Verification items for the finished model (mm, model axes). Face numbers are marked on the shaded views. A direction names the side the tool comes from. Coordinates: 2 decimals unless noted, no trailing zeros. Loops run counter-clockwise (first coordinate to the right, second up) from the corner with the lowest first, then second, coordinate; pieces in that order, holes last. Notation, with made-up numbers: (42, 22.25) -> (90, 22.25) arc R29 cw to (90, 49.25) -> close; hole circle Ø1 at (17, 56.25). An arc over 180 degrees is marked (long way). Answer as a JSON object with one key per item and string values. Group by question number.
Q1. Cross-section at B-B on y = 12.7. Record the boundary of the cut face in (x, z) (3 decimals).
Q2. Scan lines: L1, parallel to Z at x = 25.4, y = 28.15; L2, parallel to Z at x = 38.1, y = 29.15; L3, parallel to Y at x = 10.5, z = 23 (3 decimals). Record each from-to range of solid material in increasing order.
Q3. Set-up check for the marked faces 1 and 2: record each of +Z, -Z, +X, -X, +Y, -Y from which the full face is reachable in a straight line by a thin tool's end or side.
Q4. Cross-section at A-A on x = 6.35. Record the boundary of the cut face in (y, z) (3 decimals).
Q5. Cross-section at C-C on x = 25.4. Record the boundary of the cut face in (y, z) (3 decimals), and give its area (3 significant figures).
Q6. Gauge pin test, flat ends, axial feed: pin 1 Ø5.5 at (x, y) = (6.35, 12.7) entering from +Z (3 decimals); pin 2 Ø1.5 at (x, z) = (32.5, 45) entering from -Y. Record the tip position at first contact, or that the pin passes through.
Q7. Cross-section at D-D on x = 13. Record the boundary of the cut face in (y, z) (3 decimals).
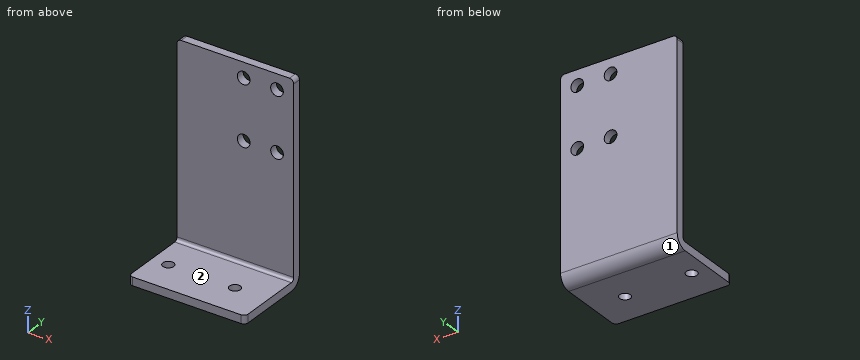
Autodesk Inventor part; units mm, degrees
ref_plane "YZ Plane" through (0, 0, 0) normal (1, 0, 0) x (0, 1, 0)
ref_plane "XZ Plane" through (0, 0, 0) normal (0, 1, 0) x (-1, 0, 0)
ref_plane "XY Plane" through (0, 0, 0) normal (0, 0, 1) x (1, 0, 0)
sketch "Sketch1" plane through (0, 0, 0) normal (0, 0, 1) x (1, 0, 0)
  line L0 (0, 0) -> (44.45, 0)
  line L1 (44.45, 0) -> (44.45, 25.4)
  line L2 (44.45, 25.4) -> (0, 25.4)
  line L3 (0, 25.4) -> (0, 0)
  circle A0 centre (6.35, 12.7) radius 2.0701
  line L4 (0, 12.7) -> (44.45, 12.7) construction
  circle A1 centre (31.75, 12.7) radius 2.0701
  dimension "d0" = 44.45
  dimension "d1" = 25.4
  dimension "d2" = 4.1402
  dimension "d6" = 25.4
  dimension "d34" = 6.35
extrude "Plate1" add sketch "Sketch1" along normal blind 3.175
sketch "Sketch2" plane through (0, 26.67, 4.445) normal (0, 1, 0) x (-1, 0, 0)
  line L0 (-44.45, 0) -> (0, 0)
  line L1 (0, 0) -> (0, 71.755)
  line L2 (0, 71.755) -> (-44.45, 71.755)
  line L3 (-44.45, 71.755) -> (-44.45, 0)
edge flange "Flange1" height 76.2 angle 90 thickness 3.175 bend radius 1.27 thickness toward (0, 1, 0) relief tear relief width 3.175 relief depth 1.5875 edges at (22.225, 25.4, 3.175) wall of the first edge with corners at (44.45, 26.67, 4.445) (0, 26.67, 4.445) (0, 26.67, 76.2) (44.45, 26.67, 76.2)
bend "Bend1"
corner "Corner1"
fillet "Fillet1" radius 1.5875 4 edges at (44.45, 0, 1.5875) (0, 0, 1.5875) (44.45, 28.2575, 76.2) (0, 28.2575, 76.2)
sketch "Sketch3" plane through (0, 26.67, 4.445) normal (0, -1, 0) x (1, 0, 0)
  line L0 (22.225, 71.755) -> (41.275, 71.755) construction
  line L1 (41.275, 71.755) -> (41.275, 37.465) construction
  line L2 (41.275, 37.465) -> (22.225, 37.465) construction
  line L3 (22.225, 37.465) -> (22.225, 71.755) construction
  circle A0 centre (38.1, 66.0019) radius 2.413
  line L4 (31.75, 71.755) -> (31.75, 37.465) construction
  line L5 (22.225, 54.61) -> (41.275, 54.61) construction
  circle A1 centre (25.4, 66.0019) radius 2.413
  circle A2 centre (38.1, 43.2181) radius 2.413
  circle A3 centre (25.4, 43.2181) radius 2.413
  line L6 (0, 70.1675) -> (0, 0)
  line L7 (42.8625, 71.755) -> (1.5875, 71.755)
  point P0 (0, -4.445)
  dimension "d23" = 34.29
  dimension "d24" = 19.05
  dimension "d27" = 4.826
  dimension "d28" = 3.175
  dimension "d29" = 5.7531
  dimension "d35" = 22.225
extrude "Extrusion1" cut sketch "Sketch3" against normal blind 25.4
equation "\"d12\" = BendReliefWidth"
equation "\"d13\" = BendReliefDepth"
equation "\"d14\" = MinimumRemnant"
equation "\"d15\" = BendRadius"
equation "\"d19\" = CornerReliefSize"
equation "\"d20\" = GapSize"
equation "\"d21\" = JacobiRadiusSize"
equation "\"BendRadius\" = Thickness"
equation "\"BendReliefWidth\" = Thickness"
equation "\"BendReliefDepth\" = 0.5 * Thickness"
equation "\"CornerReliefSize\" = 4 * Thickness"
equation "\"MinimumRemnant\" = 2 * Thickness"
equation "\"TransitionRadius\" = BendRadius"
equation "\"JacobiRadiusSize\" = BendRadius"
equation "\"GapSize\" = Thickness"
equation "\"d11\" = BendRadius"
properties part number "Pneumatic Piston Back Flange (Lt Custom)"
Computed values:
{
 "1": {"outline": "(0, 0) -> (4.28, 0) -> (4.28, 3.175) -> (0, 3.175) -> close; (8.42, 0) -> (29.68, 0) -> (29.68, 3.175) -> (8.42, 3.175) -> close; (33.82, 0) -> (44.45, 0) -> (44.45, 3.175) -> (33.82, 3.175) -> close"},
 "2": {"L1": "z = 0.95 to 45.25, 50.08 to 68.03, 72.86 to 76.2", "L2": "z = 2.06 to 45.25, 50.08 to 68.03, 72.86 to 76.2", "L3": "y = 26.67 to 29.845"},
 "3": {"face 1": "-Z, +X, -X, +Y", "face 2": "+Z, +X, -X, -Y"},
 "4": {"outline": "(0, 0) -> (10.63, 0) -> (10.63, 3.175) -> (0, 3.175) -> close; (14.77, 0) -> (25.4, 0) arc R4.445 ccw to (29.845, 4.445) -> (29.845, 76.2) -> (26.67, 76.2) -> (26.67, 4.445) arc R1.27 cw to (25.4, 3.175) -> (14.77, 3.175) -> close"},
 "5": {"outline": "(0, 0) -> (25.4, 0) arc R4.445 ccw to (29.845, 4.445) -> (29.845, 45.25) -> (26.67, 45.25) -> (26.67, 4.445) arc R1.27 cw to (25.4, 3.175) -> (0, 3.175) -> close; (26.67, 50.076) -> (29.845, 50.076) -> (29.845, 68.034) -> (26.67, 68.034) -> close; (26.67, 72.86) -> (29.845, 72.86) -> (29.845, 76.2) -> (26.67, 76.2) -> close", "area": "292 mm²"},
 "6": {"pin 1": "stops at z = 3.175", "pin 2": "stops at y = 26.67"},
 "7": {"outline": "(0, 0) -> (25.4, 0) arc R4.445 ccw to (29.845, 4.445) -> (29.845, 76.2) -> (26.67, 76.2) -> (26.67, 4.445) arc R1.27 cw to (25.4, 3.175) -> (0, 3.175) -> close"}
}
